from build123d import *

# Parameters (mm, degrees)
F1_DEPTH = 280
F3_DEPTH = 287
F4_T     = -1.2


with BuildPart() as f1:
    # F0 (on Front) → F1 (new body)
    with BuildSketch(Plane.XZ):
        Polygon((-9.899495, 9.899495), (-9.899495, -9.899495), (9.899495, -9.899495), align=None)
    extrude(amount=F1_DEPTH)

    # F2 (on face) → F3 (cut)
    with BuildSketch(Plane(origin=(0, 0, 0), x_dir=(-1, 0, 0), z_dir=(0, 1, 0))):
        Polygon((9.899495, 4.242641), (-4.242641, -9.899495), (9.899495, -9.899495), align=None)
    extrude(amount=-F3_DEPTH, mode=Mode.SUBTRACT)

    # F4
    f4_openings = [f1.faces().sort_by_distance(p)[0] for p in [
        (-2.828427, -140, -2.828427),
    ]]
    offset(amount=F4_T, openings=f4_openings)


solid = f1.part
Design review of the part built by this model. Coordinates are the model's own, in mm. A direction names the side the tool comes from. Round coordinates to 2 decimals unless told otherwise and drop trailing zeros. Loops run counter-clockwise (first coordinate to the right, second up) from the corner with the lowest first, then second, coordinate; pieces in that order, holes last. Notation, with made-up numbers: M -11.75,-31.5 L 9.25,-31.5 A25 cw 9.25,-12.5 Z; hole C 88.25,42 d10. An arc over 180 degrees is marked long. Answer as a JSON object with one key per item and string values.
Item 1: Machinability: for faces 5 (the flat face through (-9.147, -139.347, 3.49)), 6 (the flat face through (-2, -278.8, -1)), which of the approach directions +Z, -Z, +X, -X, +Y, -Y give a long, thin tool a straight path to every point of the face, cutting with its end or side? Answer none if there is none.
Answer sheet:
{"face 5": "-Z, -X, +Y, -Y", "face 6": "none"}
Item 2: The part is to be moulded in two halves that separate along Z. For faces 1 (the flat face through (-2, -1.2, -1)), 2 (the flat face through (0, -138, 0)), 3 (the flat face through (-0.739, -138.057, -0.958)), 4 (the flat face through (-9.899, -138, 7)), say which applies: pulls with the +Z half, pulls with the -Z half, needs draft (parallel to the pull), parting line crosses it, or undercut.
Answer sheet:
{"face 1": "undercut", "face 2": "pulls with the +Z half", "face 3": "undercut", "face 4": "needs draft"}
Item 3: We need section A-A on y = -52. Give the boundary of the cut face in (x, z).
Answer sheet:
{"outline": "M -9.9,4.24 L -8.7,3.04 L -8.7,7 L 7,-8.7 L 3.04,-8.7 L 4.24,-9.9 L 9.9,-9.9 L -9.9,9.9 Z"}
Item 4: We need section B-B on z = -6. Give the boundary of the cut face in (x, y).
Answer sheet:
{"outline": "M 0.34,-280 L 6,-280 L 6,0 L 0.34,0 L 0.34,-1.2 L 4.3,-1.2 L 4.3,-278.8 L 0.34,-278.8 Z"}
Item 5: Clearance check with flat-ended pins moving along their axes: P1, Ø8, axis at x = -0.5, y = -36.5, coming from the -Z side; P2, Ø1.5, axis at x = 3.5, y = -219, coming from the +Z side; P3, Ø3, axis at x = 6.5, z = -3, coming from the +Y side; P4, Ø1, axis at x = -5, y = -123, coming from the -Z side. State where each tip first meets the part, or that it passes through.
Answer sheet:
{"P1": "stops at z = -9.16", "P2": "stops at z = -2.75", "P3": "passes through", "P4": "stops at z = 2.8"}
Item 6: Wall thickness on L1, parallel to Y at x = -7.5, z = 3.5; L2, parallel to X at y = -220.5, z = 6.5; L3, parallel to X at y = -14, z = 4.25: over which ranges is each line inside the solid? List them lowest first. Write a range as from..to.
Answer sheet:
{"L1": "y = -280..-278.8, -1.2..0", "L2": "x = -9.9..-8.7, -8.2..-6.5", "L3": "x = -9.9..-8.7, -5.95..-4.25"}
